Here's the drawing with two shaded views (mm, measured from the low corner). I have some questions. A direction names the side the tool comes from. Coordinates: 2 decimals unless noted, no trailing zeros. Write each loop counter-clockwise with the first axis right and the second up, starting at its lowest first coordinate (ties: lowest second). Pieces come first, ordered by that corner, then holes.
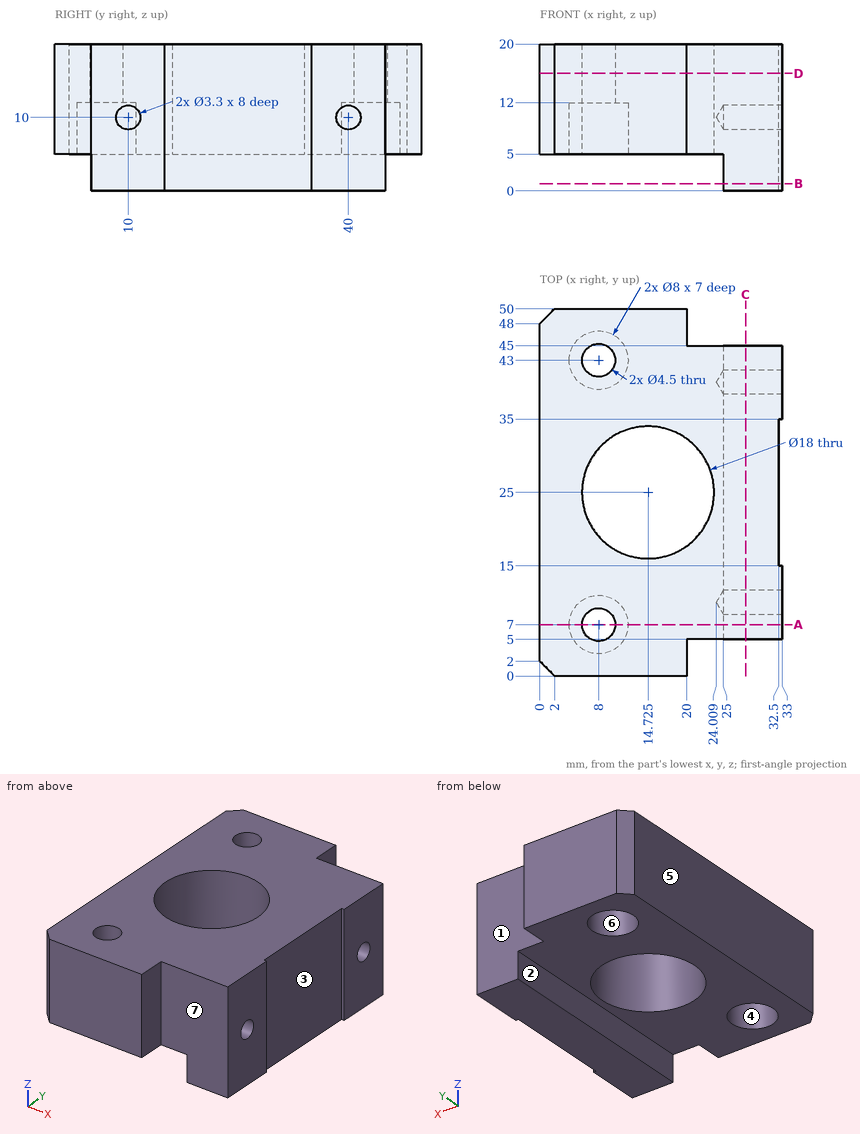
1. I want a section at A-A on y = 7. Please give me the cut outline in (x, z), plus the area to 3 significant figures.
Verdict:
outline: (0, 5) - (4, 5) - (4, 12) - (5.75, 12) - (5.75, 20) - (0, 20) - close; (10.25, 12) - (12, 12) - (12, 5) - (25, 5) - (25, 0) - (33, 0) - (33, 20) - (10.25, 20) - close
area: 443 mm2
2. I want a section at B-B on z = 1. Please give me the cut outline in (x, y), plus the area to 3 significant figures.
Verdict:
outline: (25, 5) - (33, 5) - (33, 15) - (32.5, 15) - (32.5, 35) - (33, 35) - (33, 45) - (25, 45) - close
area: 310 mm2
3. For pin 1 (1 mm diameter, centred on x = 25.5, z = 7.5, fed in from -Y); pin 2 (4 mm diameter, centred on x = 9, y = 8.5, fed in from -Z); pin 3 (4 mm diameter, centred on y = 2.5, z = 11.5, fed in from +X); pin 4 (2.5 mm diameter, centred on x = 8, y = 43, fed in from -Z), each with a flat end and sliding along its axis, tell me the tip position at first contact or that it passes through.
Verdict:
pin 1: stops at y = 5
pin 2: stops at z = 12
pin 3: stops at x = 20
pin 4: passes through
4. If we mould it in two halves opening along Y, with no side actions, what happens to the marked faces 5, 6 and 7? For each: pulls with the +Y half, pulls with the -Y half, needs draft (parallel to the pull), parting line crosses it, or undercut.
Verdict:
face 5: needs draft
face 6: undercut
face 7: pulls with the -Y half
5. I want a section at C-C on x = 28. Please give me the cut outline in (y, z), plus the area to 3 significant figures.
Verdict:
outline: (5, 0) - (45, 0) - (45, 20) - (5, 20) - close; hole circle Ø3.3 at (10, 10); hole circle Ø3.3 at (40, 10)
area: 783 mm2
6. Please list where these lines run through material, in increasing order: line 1 along Z through (x, y) = (29.75, 40); line 2 along Y through (x, z) = (5.5, 10.5); line 3 along Z through (x, y) = (7, 13.5).
Verdict:
line 1: z = 0 to 8.35, 11.65 to 20
line 2: y = 0 to 3.88, 10.12 to 39.88, 46.12 to 50
line 3: z = 5 to 20
7. On a 3-axis mill with a long thin cutter (end or side, diameter ignored), from which of +Z, -Z, +X, -X, +Y, -Y can I reach the whole of each face in a straight line? I mean the marked faces 1, 2, 3 and 4. Say none if no direction works.
Verdict:
face 1: +Z, -Z, +X, +Y
face 2: -Z, -X, +Y, -Y
face 3: +Z, -Z, +X
face 4: -Z
8. I want a section at D-D on z = 16. Give the number of separate pieces and of enclosed holes in the cut face, plus the area to 3 significant figures.
Verdict:
separate pieces: 1
enclosed holes: 3
area: 1,220 mm2
